Verification items for the finished model (mm, model axes). Face numbers are marked on the shaded views. A direction names the side the tool comes from. Give positions to 0.01 mm unless a question says otherwise; leave off trailing zeros. Write each loop counter-clockwise with the first axis right and the second up, starting at its lowest first coordinate (ties: lowest second). Pieces come first, ordered by that corner, then holes. Notation, with made-up numbers: (32, 33) -> (57, 33) arc R22 ccw to (57, 48) -> close; hole circle Ø10 at (59, 13). An arc over 180 degrees is marked (long way). Write item = value, one per line.
from build123d import *

# Parameters (mm, degrees)
F1_DEPTH = 152.4
F3_DEPTH = 80.772


with BuildPart() as f1:
    # F0 (on Right) → F1 (new body)
    with BuildSketch(Plane.YZ):
        Polygon((0, 50.8), (0, 0), (76.2, 0), (76.2, 50.8), (50.8, 50.8), (50.8, 38.1), (63.5, 38.1), (63.5, 25.4), (12.7, 25.4), (12.7, 38.1), (25.4, 38.1), (25.4, 50.8), align=None)
    extrude(amount=F1_DEPTH)

    # F2 (on face) → F3 (cut)
    with BuildSketch(Plane.XZ):
        Polygon((25.4, 12.7), (38.1, 0), (114.3, 0), (127, 12.7), align=None)
    extrude(amount=-F3_DEPTH, mode=Mode.SUBTRACT)


solid = f1.part
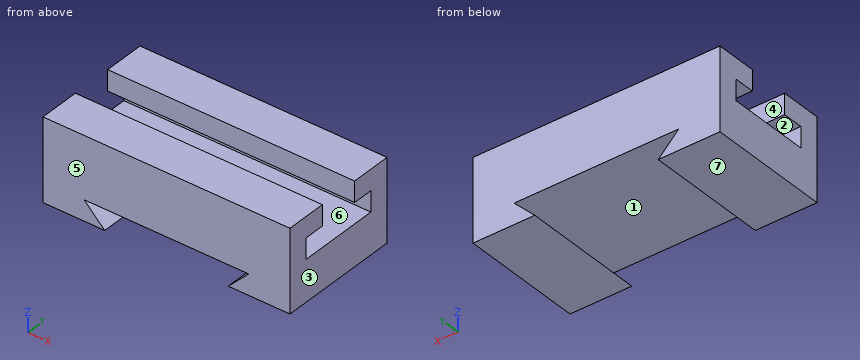
Item 1: Sectioned sample at C-C on x = 36. Record the cut outline in (y, z), then the cut area to 3 significant figures.
Response values:
outline = (0, 0) -> (76.2, 0) -> (76.2, 2.1) -> (0, 2.1) -> close; (0, 12.7) -> (76.2, 12.7) -> (76.2, 50.8) -> (50.8, 50.8) -> (50.8, 38.1) -> (63.5, 38.1) -> (63.5, 25.4) -> (12.7, 25.4) -> (12.7, 38.1) -> (25.4, 38.1) -> (25.4, 50.8) -> (0, 50.8) -> close
area = 2,100 mm^2
Item 2: Material ranges on line 1 (Y direction, x = 106.5, z = 25.5); line 2 (Z direction, x = 108.5, y = 18); line 3 (Z direction, x = 22, y = 25), recorded low to high.
Response values:
line_1 = 0 to 12.7, 63.5 to 76.2
line_2 = 12.7 to 25.4, 38.1 to 50.8
line_3 = 0 to 25.4, 38.1 to 50.8
Item 3: Mould release check, pull along Z, two halves, no side actions. Record for the marked faces 5, 6 and 7: +Z half, -Z half, draft (parallel to the pull), parting line (faces both ways), or undercut.
Response values:
face_5 = draft
face_6 = undercut
face_7 = -Z half
Item 4: Go/stop test with flat-tipped pins: P1, Ø3, axis at x = 32, y = 31.5, coming from the +Z side; P2, Ø10, axis at x = 93, y = 17.5, coming from the -Z side; P3, Ø6, axis at y = 46.5, z = 31, coming from the +X side. Record where each tip stops, or that it passes through.
Response values:
P1 = 25.4
P2 = 12.7
P3 = through
Item 5: Sectioned sample at B-B on y = 17. Record the cut outline in (x, z), then the cut area to 3 significant figures.
Response values:
outline = (0, 0) -> (38.1, 0) -> (25.4, 12.7) -> (127, 12.7) -> (114.3, 0) -> (152.4, 0) -> (152.4, 25.4) -> (0, 25.4) -> close; (0, 38.1) -> (152.4, 38.1) -> (152.4, 50.8) -> (0, 50.8) -> close
area = 4,680 mm^2
Item 6: Sectioned sample at D-D on z = 5. Record the cut outline in (x, y).
Response values:
outline = (0, 0) -> (33.1, 0) -> (33.1, 76.2) -> (0, 76.2) -> close; (119.3, 0) -> (152.4, 0) -> (152.4, 76.2) -> (119.3, 76.2) -> close
Item 7: Set-up check for the marked faces 1, 2, 3 and 4: record each of +Z, -Z, +X, -X, +Y, -Y from which the full face is reachable in a straight line by a thin tool's end or side.
Response values:
face_1 = +Y, -Y
face_2 = +X, -X
face_3 = +Z, -Z, +X, +Y, -Y
face_4 = +Z, +X, -X
Item 8: Sectioned sample at A-A on z = 27. Record the cut outline in (x, y), then the cut area to 3 significant figures.
Response values:
outline = (0, 0) -> (152.4, 0) -> (152.4, 12.7) -> (0, 12.7) -> close; (0, 63.5) -> (152.4, 63.5) -> (152.4, 76.2) -> (0, 76.2) -> close
area = 3,870 mm^2
